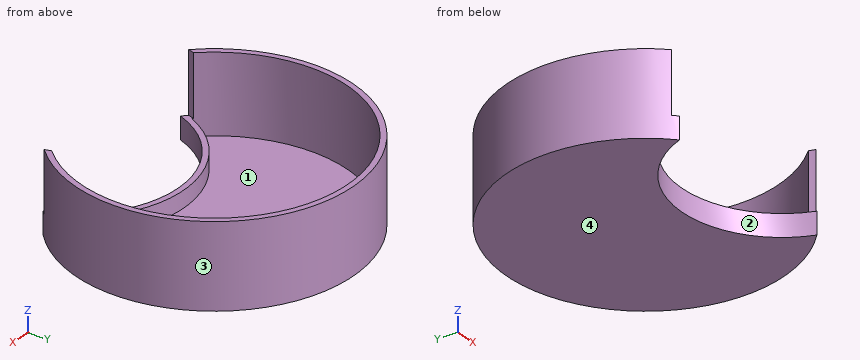
```python
from build123d import *

# Parameters (mm, degrees)
F0_R     = 63.5
F1_DEPTH = 2.54
F2_R     = 45.7677355117
F3_DEPTH = 25.4
F4_DEPTH = 12.7
F5_DEPTH = 25.4
F6_T     = -2.54
F8_R     = 46.8709431216
F9_DEPTH = 177.8


with BuildPart() as f1:
    # F0 (on Top) → F1 (new body)
    with BuildSketch(Plane.XY):
        Circle(F0_R)
    extrude(amount=F1_DEPTH)

    # F2 (on Top) → F3 (cut)
    with BuildSketch(Plane.XY):
        with Locations((0, -62.0349124074)):
            Circle(F2_R)
    extrude(amount=F3_DEPTH, mode=Mode.SUBTRACT)

    # F1_face (on face) → F4 (join)
    with BuildSketch(Plane(origin=(0, 12.1231613089, 2.54), x_dir=(1, 0, 0), z_dir=(0, 0, 1))):
        with BuildLine():
            ThreePointArc((-43.0987599006, -58.7573429253), (0, -28.3903382046), (43.0987599006, -58.7573429253))
            ThreePointArc((43.0987599006, -58.7573429253), (0, 51.3768386911), (-43.0987599006, -58.7573429253))
        make_face()
    extrude(amount=-F4_DEPTH)

    # F1_face (on face) → F5 (join)
    with BuildSketch(Plane(origin=(0, 12.1231613089, 2.54), x_dir=(1, 0, 0), z_dir=(0, 0, 1))):
        with BuildLine():
            ThreePointArc((-43.0987599006, -58.7573429253), (0, -28.3903382046), (43.0987599006, -58.7573429253))
            ThreePointArc((43.0987599006, -58.7573429253), (0, 51.3768386911), (-43.0987599006, -58.7573429253))
        make_face()
    extrude(amount=F5_DEPTH)

    # F6
    f6_openings = [f1.faces().sort_by_distance(p)[0] for p in [
        (0, 12.123161, 27.94),
    ]]
    offset(amount=F6_T, openings=f6_openings)

    # F8 (on face) → F9 (cut)
    with BuildSketch(Plane.XY):
        with Locations((0, -56.5915703773)):
            Circle(F8_R)
    extrude(amount=F9_DEPTH, mode=Mode.SUBTRACT)


solid = f1.part
```
Could you check a few things on this model? Use its own coordinates, in mm. Face numbers are marked on the shaded views. Round coordinates to 2 decimals unless told otherwise and drop trailing zeros. Loops run counter-clockwise (first coordinate to the right, second up) from the corner with the lowest first, then second, coordinate; pieces in that order, holes last. Notation, with made-up numbers: M -27,-11 L -7,-11 A31 cw -7,16 Z; hole C 28.25,69.25 d2. An arc over 180 degrees is marked long. Answer as CSV lines item,"result".
1) For pin 1 Ø4 at (x, z) = (-50, 20) entering from -Y; pin 2 Ø3 at (x, z) = (32.5, 22) entering from -Y; pin 3 Ø8 at (x, z) = (-21.5, 8.5) entering from -Y, each with a flat end and sliding along its axis, tell me the tip position at first contact or that it passes through.
From the geometry:
pin 1,"y = -41.57"
pin 2,"y = 50.6"
pin 3,"y = 55.37"
2) We'd pull the mould along X, two halves only. Please class the marked faces 1, 2, 3 and 4: released by +X, released by -X, zero draft, split by the parting line, or undercut.
From the geometry:
face 1,"undercut"
face 2,"undercut"
face 3,"split by the parting line"
face 4,"zero draft"
3) If I drill on probe 1 along X at (y, z) = (1, 13); probe 2 along X at (y, z) = (-26, -1.5); probe 3 along X at (y, z) = (0, 16), over which ranges is the centre line in solid material (lowest first)?
From the geometry:
probe 1,"-63.49 to -60.95, 60.95 to 63.49"
probe 2,"-57.93 to -55.14, -32.17 to -28.22, 28.22 to 32.17, 55.14 to 57.93"
probe 3,"-63.5 to -60.96, 60.96 to 63.5"
4) Imagine slicing it at B-B on z = -3.5. List the corners of the cut face in (x, y) for me.
From the geometry:
outline,"M -43.1,-46.63 A45.77 cw 43.1,-46.63 A63.5 ccw long Z; hole M -44.03,-42.16 A48.31 cw 44.03,-42.16 A60.96 ccw long Z"
5) Imagine slicing it at A-A on y = 0. List the corners of the cut face in (x, z) for me, and give its area (3 significant figures).
From the geometry:
outline,"M -63.5,-10.16 L 63.5,-10.16 L 63.5,27.94 L 60.96,27.94 L 60.96,-7.62 L -60.96,-7.62 L -60.96,27.94 L -63.5,27.94 Z"
area,"503 mm^2"
6) Imagine slicing it at D-D on z = 17. List the corners of the cut face in (x, y) for me.
From the geometry:
outline,"M -45.29,-44.51 A46.87 cw -44.45,-41.72 A60.96 cw long 44.45,-41.72 A46.87 cw 45.29,-44.51 A63.5 ccw long Z"
7) Imagine slicing it at C-C on x = 0. List the corners of the cut face in (y, z) for me.
From the geometry:
outline,"M -16.27,-10.16 L 63.5,-10.16 L 63.5,27.94 L 60.96,27.94 L 60.96,-7.62 L -13.73,-7.62 L -13.73,0 L -16.27,0 Z"
